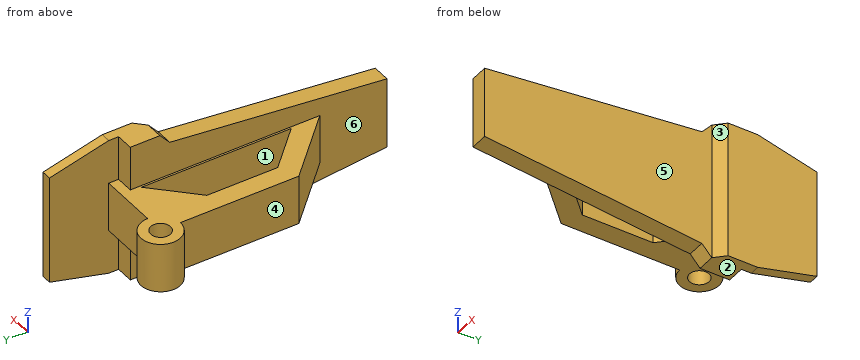
```python
from build123d import *

# Parameters (mm, degrees)
EXTRUDE_1_DEPTH          = 2.5
EXTRUDE_1_DEPTH_BACK     = 2.5
SKETCH_1_R               = 2
EXTRUDE_2_DEPTH          = 3
SKETCH_4_W               = 5
SKETCH_4_H               = 21
EXTRUDE_3_DEPTH          = 1.8
CUT_EXTRUDE_1_DEPTH      = 72.103790411
CUT_EXTRUDE_1_DEPTH_BACK = 72.103790411
CUT_EXTRUDE_2_DEPTH      = 30.885943266
CUT_EXTRUDE_3_DEPTH      = 10
SKETCH_8_R               = 1
CUT_EXTRUDE_4_DEPTH      = 70.182991672


with BuildPart() as part:
    # Sketch 1 → Extrude 1 (new, two sides: drawn at the far end of the back side and taken through both)
    # profile 1 of 2: a face of its own
    with BuildSketch(Plane.XY.offset(-EXTRUDE_1_DEPTH_BACK)):
        with Locations((54.288432405, 0.720527774)):
            Circle(SKETCH_1_R)
    # profile 2 of 2: a face of its own
    with BuildSketch(Plane.XY.offset(-EXTRUDE_1_DEPTH_BACK)):
        Polygon((54.288432405, 0.720527774), (62.288432405, 0.720527774), (62.288432405, -13.279472226), (62.288432405, -21.279472226), (54.288432405, -13.279472226), align=None)
        Polygon((56.288432405, -12.451045101), (60.288432405, -16.451045101), (60.288432405, -13.279472226), (60.288432405, -1.279472226), (56.288432405, -5.279472226), align=None, mode=Mode.SUBTRACT)
    extrude(amount=EXTRUDE_1_DEPTH + EXTRUDE_1_DEPTH_BACK)

    # Sketch 2 → Extrude 2 (add)
    with BuildSketch(Plane(origin=(62.288432405, 0, 0), x_dir=(0, 0, -1), z_dir=(1, 0, 0))):
        Polygon((-7, -3.279472226), (-4.5, -27.279472226), (4.5, -27.279472226), (7, -3.279472226), (7, 8.720527774), (-7, 8.720527774), align=None)
    extrude(amount=EXTRUDE_2_DEPTH)

    # Sketch 4 → Extrude 3 (add)
    with BuildSketch(Plane.ZY.offset(-62.288432405)):
        Polygon((-2.5, -0.279472226), (-7, -0.279472226), (-7, -3.279472226), (-4.5, -27.279472226), (4.5, -27.279472226), (7, -3.279472226), (7, -0.279472226), (2.5, -0.279472226), (2.5, -21.279472226), (-2.5, -21.279472226), align=None)
        with Locations((0, -10.779472226)):
            Rectangle(SKETCH_4_W, SKETCH_4_H)
    extrude(amount=EXTRUDE_3_DEPTH)

    # Sketch 5 → Cut-Extrude 1 (cut, two sides: drawn at the far end of the back side and taken through both)
    with BuildSketch(Plane.XY.offset(-CUT_EXTRUDE_1_DEPTH_BACK)):
        Polygon((62.288432405, -27.279472226), (62.288432405, -3.279472226), (63.288432405, -2.279472226), (63.288432405, 6.720527774), (62.288432405, 6.720527774), (62.288432405, 8.720527774), (65.288432405, 8.720527774), (65.288432405, -27.279472226), align=None)
    extrude(amount=CUT_EXTRUDE_1_DEPTH + CUT_EXTRUDE_1_DEPTH_BACK, mode=Mode.SUBTRACT)

    # Sketch 6 → Cut-Extrude 2 (cut, through all)
    with BuildSketch(Plane(origin=(62.288432405, 0, 0), x_dir=(0, 0, -1), z_dir=(1, 0, 0))):
        Polygon((-5.890422624, -4.279472226), (-3.598755957, -26.279472226), (3.598755957, -26.279472226), (5.890422624, -4.279472226), (7, -3.279472226), (4.5, -27.279472226), (-4.5, -27.279472226), (-7, -3.279472226), align=None)
    extrude(amount=-CUT_EXTRUDE_2_DEPTH, mode=Mode.SUBTRACT)

    # Sketch 7 → Cut-Extrude 3 (cut)
    with BuildSketch(Plane(origin=(63.288432405, 0, 0), x_dir=(0, 0, -1), z_dir=(1, 0, 0))):
        Polygon((-7, 0.720527774), (-5.5, 6.720527774), (-7, 6.720527774), align=None)
        Polygon((5.5, 6.720527774), (7, 6.720527774), (7, 0.720527774), align=None)
    extrude(amount=-CUT_EXTRUDE_3_DEPTH, mode=Mode.SUBTRACT)

    # Sketch 8 → Cut-Extrude 4 (cut, through all)
    with BuildSketch(Plane.XY.offset(2.5)):
        with Locations((54.288432405, 0.720527774)):
            Circle(SKETCH_8_R)
    extrude(amount=-CUT_EXTRUDE_4_DEPTH, mode=Mode.SUBTRACT)


solid = part.part
```
Source: CAD feature listing. Evaluate the final solid. Frame: model axes, mm. Face numbers are marked on the shaded views. A direction names the side the tool comes from. Coordinates: 2 decimals unless noted, no trailing zeros. Loops run counter-clockwise (first coordinate to the right, second up) from the corner with the lowest first, then second, coordinate; pieces in that order, holes last. Notation, with made-up numbers: (-12, 80.25) - (12, 80.25) arc R28 cw to (12, 115.25) - close; hole circle Ø2 at (82, 8). An arc over 180 degrees is marked (long way). Answer as CSV lines item,"result".
1. Section C-C (z = 1.25). Return loops of the section in (x, y).
Established:
outline,"(54.29, -13.28) - (60.49, -19.48) - (60.49, -26.28) - (62.29, -26.28) - (62.29, -3.28) - (63.29, -2.28) - (63.29, 6.72) - (62.29, 6.72) - (62.29, 0.72) - (56.29, 0.72) arc R2 ccw (long way) to (54.29, -1.28) - close; hole circle Ø2 at (54.29, 0.72); hole (56.29, -12.45) - (60.29, -16.45) - (60.29, -1.28) - (56.29, -5.28) - close"
2. Section D-D (z = -3.25). Return loops of the section in (x, y), then the cut area to 3 significant figures.
Established:
outline,"(60.49, -26.28) - (62.29, -26.28) - (62.29, -3.28) - (63.29, -2.28) - (63.29, 6.72) - (62.29, 6.72) - (62.29, -0.28) - (60.49, -0.28) - close"
area,"56.3 mm2"
3. Ray query, line 1 (X direction, y = -7, z = 0.25); line 2 (Y direction, x = 54.25, z = -1); line 3 (X direction, y = 5, z = -5.5). Return the intervals inside material, ascending.
Established:
line 1,"x = 54.29 to 56.29, 60.29 to 62.29"
line 2,"y = -1.28 to -0.28, 1.72 to 2.72"
line 3,"x = 62.29 to 63.29"
4. Reachability of the marked faces 4, 5 and 6 from +Z, -Z, +X, -X, +Y, -Y: full face, straight path, thin tool, end or side. Return the list, or none.
Established:
face 4,"+Z, -Z, -X, -Y"
face 5,"+Z, -Z, +X, -Y"
face 6,"-X, -Y"
5. Contact query for flat-ended pins moving along their axis: pin 1 (2 mm diameter, centred on y = 3.5, z = -2.5, fed in from -X); pin 2 (5 mm diameter, centred on x = 57, z = 2.5, fed in from -Y); pin 3 (7 mm diameter, centred on y = -15, z = 3.5, fed in from +X); pin 4 (1.8 mm diameter, centred on x = 54.29, y = 0.72, fed in from -Z). Output: stop coordinate, or through.
Established:
pin 1,"stops at x = 53.38"
pin 2,"stops at y = -18.49"
pin 3,"stops at x = 62.29"
pin 4,"passes through"
6. Mould query, pull axis Y, two halves, no side actions, for the marked faces 1, 2 and 3. Classes: released by +Y, released by -Y, zero draft, split by the parting line, or undercut.
Established:
face 1,"undercut"
face 2,"zero draft"
face 3,"released by -Y"
7. Section B-B (y = -15). Return loops of the section in (x, z).
Established:
outline,"(56.01, -2.5) - (58.84, -2.5) - (58.84, 2.5) - (56.01, 2.5) - close; (60.29, -2.5) - (60.49, -2.5) - (60.49, -4.77) - (62.29, -4.77) - (62.29, 4.77) - (60.49, 4.77) - (60.49, 2.5) - (60.29, 2.5) - close"
8. Section A-A (x = 57.75). Return loops of the section in (y, z).
Established:
outline,"(-16.74, -2.5) - (-13.91, -2.5) - (-13.91, 2.5) - (-16.74, 2.5) - close; (-3.82, -2.5) - (0.72, -2.5) - (0.72, 2.5) - (-3.82, 2.5) - close"
